from build123d import *

# Parameters (mm, degrees)
SKETCH1_R              = 2.4765
BOSS_EXTRUDE1_DEPTH    = 6.35
SKETCH2_R              = 6.477
CUT_EXTRUDE1_DEPTH     = 3.175
SKETCH3_R              = 4.318
SKETCH3_R_2            = 2.4765
BOSS_EXTRUDE2_DEPTH    = 6.35
SKETCH4_R              = 4.445
SKETCH4_R_2            = 2.4765
BOSS_EXTRUDE3_DEPTH    = 13.335
SKETCH6_R              = 3.175
CUT_EXTRUDE2_DEPTH     = 1.27
F_10_24_TAPPED_HOLE1_D = 3.7973


with BuildPart() as part:
    # Sketch1 → Boss-Extrude1 (new body)
    with BuildSketch(Plane(origin=(0, 0, 0), x_dir=(1, 0, 0), z_dir=(0, 1, 0))):
        with BuildLine():
            Line((0, 12.7), (-43.815, 12.7))
            ThreePointArc((-43.815, 12.7), (-46.06006403, 11.77006403), (-46.99, 9.525))
            Line((-46.99, 9.525), (-46.99, -9.525))
            ThreePointArc((-46.99, -9.525), (-46.06006403, -11.77006403), (-43.815, -12.7))
            Line((-43.815, -12.7), (0, -12.7))
            ThreePointArc((0, -12.7), (6.475754782, -10.924953089), (11.141309797, -6.096))
            ThreePointArc((11.141309797, -6.096), (12.307698551, -4.888761728), (13.926637247, -4.445))
            Line((13.926637247, -4.445), (40.683362753, -4.445))
            ThreePointArc((40.683362753, -4.445), (42.302301449, -4.888761728), (43.468690203, -6.096))
            ThreePointArc((43.468690203, -6.096), (67.31, 0), (43.468690203, 6.096))
            ThreePointArc((43.468690203, 6.096), (42.302301449, 4.888761728), (40.683362753, 4.445))
            Line((40.683362753, 4.445), (13.926637247, 4.445))
            ThreePointArc((13.926637247, 4.445), (12.307698551, 4.888761728), (11.141309797, 6.096))
            ThreePointArc((11.141309797, 6.096), (6.475754782, 10.924953089), (0, 12.7))
        make_face()
        with Locations(Location((0, 0, 0), (0, 0, 270))):
            Circle(SKETCH1_R, mode=Mode.SUBTRACT)
        with Locations(Location((54.61, 0, 0), (0, 0, 270))):
            Circle(SKETCH1_R, mode=Mode.SUBTRACT)
    extrude(amount=BOSS_EXTRUDE1_DEPTH)

    # Sketch2 → Cut-Extrude1 (cut)
    with BuildSketch(Plane(origin=(0, 6.35, 0), x_dir=(1, 0, 0), z_dir=(0, 1, 0))):
        with Locations(Location((0, 0, 0), (0, 0, 270))):
            Circle(SKETCH2_R)
    extrude(amount=-CUT_EXTRUDE1_DEPTH, mode=Mode.SUBTRACT)

    # Sketch3 → Boss-Extrude2 (add)
    with BuildSketch(Plane(origin=(0, 3.175, 0), x_dir=(1, 0, 0), z_dir=(0, 1, 0))):
        with Locations(Location((0, 0, 0), (0, 0, 270))):
            Circle(SKETCH3_R)
        with Locations(Location((0, 0, 0), (0, 0, 270))):
            Circle(SKETCH3_R_2, mode=Mode.SUBTRACT)
    extrude(amount=BOSS_EXTRUDE2_DEPTH)

    # Sketch4 → Boss-Extrude3 (add)
    with BuildSketch(Plane(origin=(0, 6.35, 0), x_dir=(1, 0, 0), z_dir=(0, 1, 0))):
        with Locations(Location((54.61, 0, 0), (0, 0, 270))):
            Circle(SKETCH4_R)
        with Locations(Location((54.61, 0, 0), (0, 0, 270))):
            Circle(SKETCH4_R_2, mode=Mode.SUBTRACT)
    extrude(amount=BOSS_EXTRUDE3_DEPTH)

    # Sketch6 → Cut-Extrude2 (cut)
    with BuildSketch(Plane(origin=(0, 6.35, 0), x_dir=(1, 0, 0), z_dir=(0, 1, 0))):
        with Locations(Location((-40.64, 6.35, 0), (0, 0, 270))):
            Circle(SKETCH6_R)
        with Locations(Location((-40.64, -6.35, 0), (0, 0, 270))):
            Circle(SKETCH6_R)
    extrude(amount=-CUT_EXTRUDE2_DEPTH, mode=Mode.SUBTRACT)

    # #10-24 Tapped Hole1 (through all)
    with Locations(Plane(origin=(-40.64, 6.35, -6.35), x_dir=(0, 0, 1), z_dir=(0, 1, 0))):
        with Locations((0, 0), (12.7, 0)):
            Hole(F_10_24_TAPPED_HOLE1_D / 2)


solid = part.part
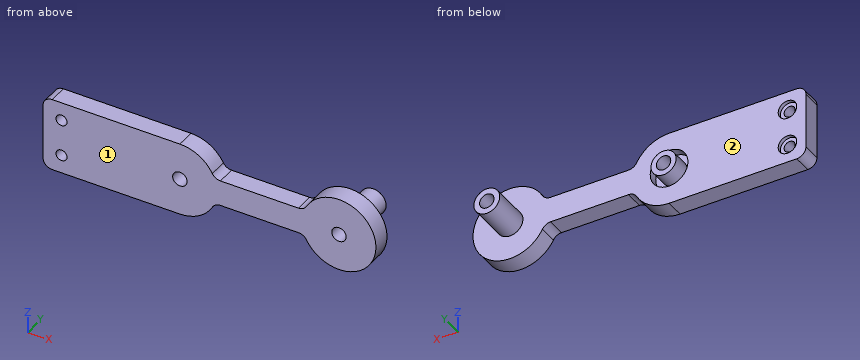
Read the model definition and answer for the solid it produces. Units are mm, in the model's axes. Face numbers are marked on the shaded views. Round coordinates to 2 decimals unless told otherwise and drop trailing zeros. Order: outer loops, then holes, each group sorted by start corner. A loop starts at its lowest first (then second) coordinate and runs counter-clockwise, first axis right, second up.
1) The part is cut by section B-B on x = -40.64. Write down the section's boundary in (y, z) (3 decimals), plus the area to 3 significant figures.
2) Straight lines are drawn through the part: L1, parallel to X at y = 10.75, z = 0 (1 decimal); L2, parallel to X at y = 3.25, z = 3; L3, parallel to X at y = 15, z = 0.25. For each, find the intervals that lie inside material, in ascending order.
3) The part is cut by section C-C on z = 11. Write down the section's boundary in (x, y).
4) Flat-ended cylindrical pins translate along their axes: pin 1 (4 mm diameter, centred on x = 2, z = -0.5, fed in from +Y) (3 decimals); pin 2 (5 mm diameter, centred on x = 14, z = -4, fed in from +Y); pin 3 (5 mm diameter, centred on y = 4.5, z = 0.5, fed in from +X); pin 4 (1 mm diameter, centred on y = 15, z = 4.5, fed in from -X). Find the tip coordinate at first contact, or state that the pin passes through.
5) The mould has two halves that part along X. Classify the marked faces 1 and 2: released by +X, released by -X, zero draft, split by the parting line, or undercut.
6) The part is cut by section D-D on y = 11. Write down the section's boundary in (x, z) (1 decimal), plus the area to 3 significant figures.
Resolved:
1. outline: (0, -12.7) - (6.35, -12.7) - (6.35, -9.525) - (5.08, -9.525) - (5.08, -8.249) - (0, -8.249) - close; (0, -4.451) - (5.08, -4.451) - (5.08, -3.175) - (6.35, -3.175) - (6.35, 3.175) - (5.08, 3.175) - (5.08, 4.451) - (0, 4.451) - close; (0, 8.249) - (5.08, 8.249) - (5.08, 9.525) - (6.35, 9.525) - (6.35, 12.7) - (0, 12.7) - close
1. area: 107 mm2
2. L1: x = 50.2 to 52.1, 57.1 to 59.1
2. L2: x = -46.99 to -5.74, -3.11 to 3.11, 5.74 to 66.95
2. L3: x = 50.17 to 52.15, 57.07 to 59.05
3. outline: (-46.63, 0) - (6.35, 0) - (6.35, 6.35) - (-46.63, 6.35) - close; (48.26, 0) - (60.96, 0) - (60.96, 6.35) - (48.26, 6.35) - close
4. pin 1: stops at y = 9.525
4. pin 2: stops at y = 6.35
4. pin 3: stops at x = 67.31
4. pin 4: stops at x = 52.67
5. face 1: zero draft
5. face 2: undercut
6. outline: circle Ø8.9 at (54.6, 0); hole circle Ø5 at (54.6, 0)
6. area: 42.8 mm2
